Geometry check sheet. Reference: the model listing, model coordinates, mm. A direction names the side the tool comes from. Round coordinates to 2 decimals unless told otherwise and drop trailing zeros. Order: outer loops, then holes, each group sorted by start corner. A loop starts at its lowest first (then second) coordinate and runs counter-clockwise, first axis right, second up. Notation, with made-up numbers: M 70,55.5 L 129,55.5 A16 ccw 129,79.5 Z; hole C 29,4.5 d5. An arc over 180 degrees is marked long. Return JSON: item names as keys, results as strings. Group by question number.
Autodesk Inventor part; units mm, degrees
ref_plane "YZ Plane" through (0, 0, 0) normal (1, 0, 0) x (0, 1, 0)
ref_plane "XZ Plane" through (0, 0, 0) normal (0, 1, 0) x (-1, 0, 0)
ref_plane "XY Plane" through (0, 0, 0) normal (0, 0, 1) x (1, 0, 0)
sketch "Sketch1" plane through (0, 0, 0) normal (0, 0, 1) x (1, 0, 0)
  circle A0 centre (0, 0) radius 25.4 construction
  circle A1 centre (0, 0) radius 19.05
  arc A2 (19.0262, -0.952) -> (10.5106, 23.1233) centre (3.175, 6.985) ccw
  arc A3 (8.7227, 16.9357) -> (10.5106, 23.1233) centre (6.8532, 20.828) ccw
  arc A4 (-10.3054, 16.0219) -> (-14.7701, 20.6641) centre (-14.611, 16.349) ccw
  arc A5 (10.3375, 16.0012) -> (-14.7701, 20.6641) centre (-4.4617, 6.2421) ccw
  arc A6 (-19.0281, -0.9138) -> (-25.2807, -2.4592) centre (-21.4642, -4.479) ccw
  arc A7 (-8.6887, 16.9532) -> (-25.2807, -2.4592) centre (-7.6367, -0.7429) ccw
  arc A8 (-8.7227, -16.9357) -> (-10.5106, -23.1233) centre (-6.8532, -20.828) ccw
  arc A9 (-19.0262, 0.952) -> (-10.5106, -23.1233) centre (-3.175, -6.985) ccw
  arc A10 (10.3054, -16.0219) -> (14.7701, -20.6641) centre (14.611, -16.349) ccw
  arc A11 (-10.3375, -16.0012) -> (14.7701, -20.6641) centre (4.4617, -6.2421) ccw
  arc A12 (19.0281, 0.9138) -> (25.2807, 2.4592) centre (21.4642, 4.479) ccw
  arc A13 (8.6887, -16.9532) -> (25.2807, 2.4592) centre (7.6367, 0.7429) ccw
  circle A14 centre (0, 0) radius 2.6035
  point P0 (9.3754, 17.3232)
  point P1 (-10.3146, 16.781)
  point P2 (-19.6901, -0.5423)
  point P3 (-9.3754, -17.3232)
  point P4 (10.3146, -16.781)
  point P5 (19.6901, 0.5423)
  dimension "d0" = 50.8
  dimension "d1" = 38.1
  dimension "d3" = 4.318
  dimension "d4" = 6.985
  dimension "d5" = 3.175
  dimension "d6" = 20.828
  dimension "d9" = 360
  dimension "d11" = 5.207
extrude "Extrusion1" add sketch "Sketch1" along normal blind 25.4 contours A1 | A1 A12 A2 | A1 A5 A3 A2 A12 | A2 A12 A13 A10 A1 | A1 A3 A5 | A10 A13 A1 | A1 A7 A4 A5 A3 | A13 A10 A11 A8 A1 | A1 A4 A7 | A8 A11 A1 | A1 A9 A6 A7 A4 | A11 A8 A9 A6 A1 | A1 A6 A9 | A14
extrude "Extrusion2" cut sketch "Sketch1" along normal through all contours A14
properties part number "THE_WHEEL"
Q1. Section check A-A on y = 19. Record the cut outline in (x, z), plus the area to 3 significant figures.
Q2. Release check for a two-part mould opening along Y. For faces 3 (the face through (-2.219, 23.827, 12.522)), 4 (the face through (2.219, -23.827, 12.522)), 5 (the face through (0, -5, 25.4)), 6 (the face through (11.808, -19.634, 12.522)) record: +Y half, -Y half, draft (parallel to the pull), parting line (faces both ways), or undercut.
Q3. Section check C-C on z = 10.25. Record the cut outline in (x, y) (1 decimal), plus the area to 3 significant figures.
Q4. Section check B-B on x = -14. Record the cut outline in (y, z).
Q5. Material ranges on line 1 along X through (y, z) = (2, 13); line 2 along Y through (x, z) = (0, 11); line 3 along X through (y, z) = (0, 13), recorded low to high.
Q6. Section check D-D on y = 7.5. Record the cut outline in (x, z).
Q7. Depth check by flat-ended pin: pin 1 Ø8 at (y, z) = (-14.5, 15) entering from -X; pin 2 Ø8 at (x, z) = (-15, 4.5) entering from +Y; pin 3 Ø8 at (y, z) = (-19, 21.5) entering from -X. Enter the tip coordinate at first touch or a pass-through.
Q8. Set-up check for faces 1 (the face through (22.91, 0.41, 12.52)), 2 (the face through (21.744, -9.992, 12.522)): record each of +Z, -Z, +X, -X, +Y, -Y from which the full face is reachable in a straight line by a thin tool's end or side.
Geometry check:
{
 "1": {"outline": "M -11.2,0 L 7.85,0 L 7.85,25.4 L -11.2,25.4 Z; M 10.77,0 L 16.21,0 L 16.21,25.4 L 10.77,25.4 Z", "area": "622 mm^2"},
 "2": {"face 3": "+Y half", "face 4": "-Y half", "face 5": "draft", "face 6": "undercut"},
 "3": {"outline": "M -25.3,-2.5 A4.3 cw -19.7,-0.5 A17.7 ccw -10.5,-23.1 A4.3 cw -9.4,-17.3 A17.7 ccw 14.8,-20.7 A4.3 cw 10.3,-16.8 A17.7 ccw 25.3,2.5 A4.3 cw 19.7,0.5 A17.7 ccw 10.5,23.1 A4.3 cw 9.4,17.3 A17.7 ccw -14.8,20.7 A4.3 cw -10.3,16.8 A17.7 ccw Z; hole C 0,0 d5.2", "area": "1,680 mm^2"},
 "4": {"outline": "M -21.02,0 L 15.8,0 L 15.8,25.4 L -21.02,25.4 Z; M 20.62,0 L 21.18,0 L 21.18,25.4 L 20.62,25.4 Z"},
 "5": {"line 1": "x = -25.15 to -1.67, 1.67 to 20.19, 25 to 25.32", "line 2": "y = -23.4 to -2.6, 2.6 to 23.4", "line 3": "x = -25.35 to -2.6, 2.6 to 25.35"},
 "6": {"outline": "M -23.33,0 L 20.89,0 L 20.89,25.4 L -23.33,25.4 Z"},
 "7": {"pin 1": "stops at x = -20.55", "pin 2": "stops at y = 22.72", "pin 3": "stops at x = -18.99"},
 "8": {"face 1": "+Z, -Z", "face 2": "+Z, -Z, +X"}
}
